from build123d import *

# Parameters (mm, degrees)
F0_R     = 24.5
F0_R_2   = 1.75
F0_W     = 6.2
F0_H     = 6.2
F1_DEPTH = 6.35
F0_R_3   = 2.3
F2_DEPTH = 4.32


with BuildPart() as f1:
    # F0 (on Top) → F1 (new body)
    with BuildSketch(Plane.XY):
        Circle(F0_R)
        with Locations((0, -18.5)):
            Circle(F0_R_2, mode=Mode.SUBTRACT)
        with Locations((-18.5, 0)):
            Circle(F0_R_2, mode=Mode.SUBTRACT)
        Rectangle(F0_W, F0_H, mode=Mode.SUBTRACT)
        with Locations((18.5, 0)):
            Circle(F0_R_2, mode=Mode.SUBTRACT)
        with Locations((0, 18.5)):
            Circle(F0_R_2, mode=Mode.SUBTRACT)
    extrude(amount=F1_DEPTH)

    # F0 (on Top) → F2 (join)
    with BuildSketch(Plane.XY):
        Rectangle(F0_W, F0_H)
        Circle(F0_R_3, mode=Mode.SUBTRACT)
    extrude(amount=F2_DEPTH)


solid = f1.part
Model file for the job. Use its own axes, mm. A direction names the side the tool comes from. Give positions to 0.01 mm unless a question says otherwise; leave off trailing zeros. Loops run counter-clockwise (first coordinate to the right, second up) from the corner with the lowest first, then second, coordinate; pieces in that order, holes last. Notation, with made-up numbers: (57.5, 17.25) -> (108.5, 17.25) arc R17 ccw to (108.5, 34.25) -> close; hole circle Ø4 at (68, 65). An arc over 180 degrees is marked (long way). Use a Markdown table: item, result. Add a question column.
(1) Wall check: line 1 along Y through (x, z) = (0, 4); line 2 along Y through (x, z) = (1.5, 5.5); line 3 along X through (y, z) = (-17, 5.5). Give the ranges that are in metal, low to high.
(2) Slice it at C-C on y = -18.5. List the corners of the cut face in (x, z).
(3) Tool access for faces 1 (the cylindrical face through (16.75, 0.08, 3.13)), 2 (the flat face through (-3.1, 0, 5)): list every direction of +Z, -Z, +X, -X, +Y, -Y with a clear straight run to the whole face (end or side of a thin tool).
(4) Slice it at D-D on z = 2.75. List the corners of the cut face in (x, y).
(5) Mould opens along X. For faces 3 (the flat face through (0, -3.1, 5)), 4 (the cylindrical face through (-20.25, 0.08, 3.13)), 5 (the cylindrical face through (13.17, 20.66, 3.13)), 6 (the flat face through (0, -5, 6.35)) say: +X half, -X half, draft (parallel to the pull), parting line (faces both ways), or undercut.
(6) Drop flat-ended pins along their axis: pin 1 Ø7 at (x, y) = (-1, 0) entering from +Z; pin 2 Ø2 at (x, z) = (1.5, 5.5) entering from +Y; pin 3 Ø0.6 at (y, z) = (0.5, 5.5) entering from -X; pin 4 Ø2 at (x, z) = (-9.5, 2.5) entering from +Y. Give the stop position or say it passes through.
(7) Slice it at A-A on y = 0. List the corners of the cut face in (x, z).
Filled sheet:
| question | item | result |
|---|---|---|
| 1 | line 1 | -24.5 to -20.25, -16.75 to -2.3, 2.3 to 16.75, 20.25 to 24.5 |
| 1 | line 2 | -24.45 to -19.4, -17.6 to -3.1, 3.1 to 17.6, 19.4 to 24.45 |
| 1 | line 3 | -17.64 to -0.9, 0.9 to 17.64 |
| 2 | outline | (-16.06, 0) -> (-1.75, 0) -> (-1.75, 6.35) -> (-16.06, 6.35) -> close; (1.75, 0) -> (16.06, 0) -> (16.06, 6.35) -> (1.75, 6.35) -> close |
| 3 | face 1 | +Z, -Z |
| 3 | face 2 | +Z |
| 4 | outline | circle Ø49 at (0, 0); hole circle Ø3.5 at (-18.5, 0); hole circle Ø4.6 at (0, 0); hole circle Ø3.5 at (0, -18.5); hole circle Ø3.5 at (0, 18.5); hole circle Ø3.5 at (18.5, 0) |
| 5 | face 3 | undercut |
| 5 | face 4 | undercut |
| 5 | face 5 | parting line |
| 5 | face 6 | draft |
| 6 | pin 1 | z = 6.35 |
| 6 | pin 2 | y = 24.49 |
| 6 | pin 3 | x = -24.5 |
| 6 | pin 4 | y = 22.98 |
| 7 | outline | (-24.5, 0) -> (-20.25, 0) -> (-20.25, 6.35) -> (-24.5, 6.35) -> close; (-16.75, 0) -> (-2.3, 0) -> (-2.3, 4.32) -> (-3.1, 4.32) -> (-3.1, 6.35) -> (-16.75, 6.35) -> close; (2.3, 0) -> (16.75, 0) -> (16.75, 6.35) -> (3.1, 6.35) -> (3.1, 4.32) -> (2.3, 4.32) -> close; (20.25, 0) -> (24.5, 0) -> (24.5, 6.35) -> (20.25, 6.35) -> close |
